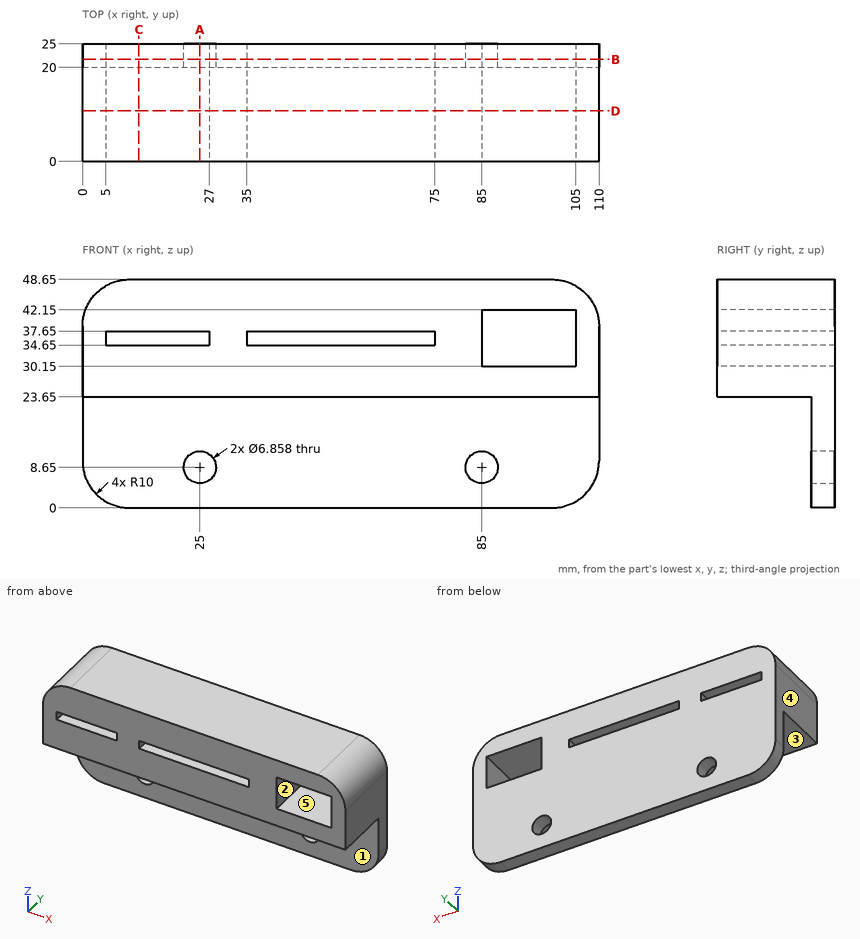
Check sheet for the drawn part. Datum: minimum x, y, z corner. Units: mm. A direction names the side the tool comes from. Coordinates: 2 decimals unless noted, no trailing zeros. Loops run counter-clockwise (first coordinate to the right, second up) from the corner with the lowest first, then second, coordinate; pieces in that order, holes last. Notation, with made-up numbers: M -5.5,14 L 43.5,14 A19 ccw 43.5,40 Z; hole C 7,50 d4. An arc over 180 degrees is marked long. Answer as a JSON object with one key per item and string values.
1. Sectioned sample at B-B on y = 21.75. Record the cut outline in (x, z).
Outcome:
{"outline": "M 0,10 A10 ccw 10,0 L 100,0 A10 ccw 110,10 L 110,38.65 A10 ccw 100,48.65 L 10,48.65 A10 ccw 0,38.65 Z; hole M 5,34.65 L 27,34.65 L 27,37.65 L 5,37.65 Z; hole C 25,8.65 d6.86; hole M 35,34.65 L 75,34.65 L 75,37.65 L 35,37.65 Z; hole C 85,8.65 d6.86; hole M 85,30.15 L 105,30.15 L 105,42.15 L 85,42.15 Z"}
2. Sectioned sample at D-D on y = 10.75. Record the cut outline in (x, z).
Outcome:
{"outline": "M 0,23.65 L 110,23.65 L 110,38.65 A10 ccw 100,48.65 L 10,48.65 A10 ccw 0,38.65 Z; hole M 5,34.65 L 27,34.65 L 27,37.65 L 5,37.65 Z; hole M 35,34.65 L 75,34.65 L 75,37.65 L 35,37.65 Z; hole M 85,30.15 L 105,30.15 L 105,42.15 L 85,42.15 Z"}
3. Scan lines: L1, parallel to X at y = 18, z = 37.5; L2, parallel to Z at x = 36, y = 21; L3, parallel to Z at x = 57, y = 19.5. Record each from-to range of solid material in increasing order. Write a range as from..to.
Outcome:
{"L1": "0..5, 27..35, 75..85, 105..110", "L2": "0..34.65, 37.65..48.65", "L3": "23.65..34.65, 37.65..48.65"}
4. Release check for a two-part mould opening along Z. For the marked faces 1, 2 and 3 record: pulls with the +Z half, pulls with the -Z half, needs draft (parallel to the pull), parting line crosses it, or undercut.
Outcome:
{"face 1": "needs draft", "face 2": "undercut", "face 3": "pulls with the -Z half"}
5. Sectioned sample at A-A on x = 25. Record the cut outline in (y, z), and give its area (3 significant figures).
Outcome:
{"outline": "M 0,23.65 L 20,23.65 L 20,12.08 L 25,12.08 L 25,34.65 L 0,34.65 Z; M 0,37.65 L 25,37.65 L 25,48.65 L 0,48.65 Z; M 20,0 L 25,0 L 25,5.22 L 20,5.22 Z", "area": "634 mm²"}
6. Depth check by flat-ended pin: P1, Ø9.5, axis at y = 10.5, z = 37, coming from the -X side; P2, Ø5.5, axis at x = 25, z = 8.65, coming from the +Y side; P3, Ø1.5, axis at x = 31, z = 10, coming from the -Y side; P4, Ø6, axis at x = 32, y = 8, coming from the -Z side. Enter the tip coordinate at first touch or a pass-through.
Outcome:
{"P1": "x = 0", "P2": "through", "P3": "y = 20", "P4": "z = 23.65"}
7. Access from +Z, -Z, +X, -X, +Y, -Y to the whole of each face (thin tool, end or side, straight path). Record for the marked faces 4 and 5.
Outcome:
{"face 4": "+Z, -Z, -X, +Y, -Y", "face 5": "+Y, -Y"}
8. Sectioned sample at C-C on x = 12. Record the cut outline in (y, z), and give its area (3 significant figures).
Outcome:
{"outline": "M 0,23.65 L 20,23.65 L 20,0 L 25,0 L 25,34.65 L 0,34.65 Z; M 0,37.65 L 25,37.65 L 25,48.65 L 0,48.65 Z", "area": "668 mm²"}
